```python
from build123d import *

# Parameters (mm, degrees)
F1_DEPTH = 22.5
F3_R     = 2.75
F4_DEPTH = 22.5


with BuildPart() as f1:
    # F0 (on Top) → F1 (new body)
    with BuildSketch(Plane.XY):
        Polygon((0, 50.875000723), (0, -13.124999277), (9.25, -13.124999277), (9.25, 22.875000723), (8.2500004293, 22.875000723), (8.2500004293, 34.875000723), (7.2500008586, 34.875000723), (7.2500008586, 50.875000723), align=None)
        Polygon((-9.25, -13.124999277), (0, -13.124999277), (0, 50.875000723), (-7.2500008586, 50.875000723), (-7.2500008586, 34.875000723), (-8.2500004293, 34.875000723), (-8.2500004293, 22.875000723), (-9.25, 22.875000723), align=None)
    extrude(amount=F1_DEPTH)

    # F3 (on offset) → F4 (cut)
    with BuildSketch(Plane(origin=(-9.25, 0, 0), x_dir=(0, -1, 0), z_dir=(-1, 0, 0))):
        with Locations((2.124999277, 11.25)):
            Circle(F3_R)
    extrude(amount=-F4_DEPTH, mode=Mode.SUBTRACT)


solid = f1.part
```
Build history of the part. All positions in model axes, mm. A direction names the side the tool comes from. Give positions to 0.01 mm unless a question says otherwise; leave off trailing zeros. Loops run counter-clockwise (first coordinate to the right, second up) from the corner with the lowest first, then second, coordinate; pieces in that order, holes last.
1) Drop flat-ended pins along their axis: P1, Ø6, axis at y = 31, z = 14.5, coming from the -X side; P2, Ø12, axis at y = 39.5, z = 10, coming from the +X side; P3, Ø1.1, axis at x = -8.5, z = 7, coming from the +Y side (3 decimals). Give the stop position or say it passes through.
Values follow:
P1: stops at x = -8.25
P2: stops at x = 8.25
P3: stops at y = 34.875
2) Band-saw the part on D-D on z = 17. List the corners of the cut face in (x, y) (3 decimals).
Values follow:
outline: (-9.25, -13.125) - (9.25, -13.125) - (9.25, 22.875) - (8.25, 22.875) - (8.25, 34.875) - (7.25, 34.875) - (7.25, 50.875) - (-7.25, 50.875) - (-7.25, 34.875) - (-8.25, 34.875) - (-8.25, 22.875) - (-9.25, 22.875) - close
3) Band-saw the part on B-B on x = 3. List the corners of the cut face in (y, z) (3 decimals), then the cut area to 3 significant figures.
Values follow:
outline: (-13.125, 0) - (50.875, 0) - (50.875, 22.5) - (-13.125, 22.5) - close; hole circle Ø5.5 at (-2.125, 11.25)
area: 1,420 mm2
4) Probe line 1 along Y through (x, z) = (7.75, 11) (3 decimals); line 2 along X through (y, z) = (31, 8.5); line 3 along Y through (x, z) = (6.5, 12) (3 decimals). List the from-to ranges inside material, lowest first.
Values follow:
line 1: y = -13.125 to -4.864, 0.614 to 34.875
line 2: x = -8.25 to 8.25
line 3: y = -13.125 to -4.771, 0.521 to 50.875
5) Two-plate mould, pull along Y, no slides. Class faces 4 (the face through (0, -13.125, 11)), 5 (the face through (-0.13, -0.1, 13.11)), 6 (the face through (0, 50.875, 11)), 7 (the face through (-7.25, 43, 11)): released by +Y, released by -Y, zero draft, split by the parting line, or undercut.
Values follow:
face 4: released by -Y
face 5: undercut
face 6: released by +Y
face 7: zero draft
6) Band-saw the part on C-C on y = 33. List the corners of the cut face in (x, z), then the cut area to 3 significant figures.
Values follow:
outline: (-8.25, 0) - (8.25, 0) - (8.25, 22.5) - (-8.25, 22.5) - close
area: 371 mm2
7) 3-axis set-ups, long thin cutter, end or side, ignore diameter. For faces 1 (the face through (-9.25, 5, 11)), 2 (the face through (7.25, 43, 11)), 3 (the face through (-8.25, 29, 11)): which of +Z, -Z, +X, -X, +Y, -Y reach the whole face in a straight line?
Values follow:
face 1: +Z, -Z, -X, +Y, -Y
face 2: +Z, -Z, +X, +Y
face 3: +Z, -Z, -X, +Y
8) Band-saw the part on A-A on z = 11.25. List the corners of the cut face in (x, y) (3 decimals), then the cut area to 3 significant figures.
Values follow:
outline: (-9.25, -13.125) - (9.25, -13.125) - (9.25, -4.875) - (-9.25, -4.875) - close; (-9.25, 0.625) - (9.25, 0.625) - (9.25, 22.875) - (8.25, 22.875) - (8.25, 34.875) - (7.25, 34.875) - (7.25, 50.875) - (-7.25, 50.875) - (-7.25, 34.875) - (-8.25, 34.875) - (-8.25, 22.875) - (-9.25, 22.875) - close
area: 994 mm2
